Verification items for the finished model (mm, model axes). Round coordinates to 2 decimals unless told otherwise and drop trailing zeros. Loops run counter-clockwise (first coordinate to the right, second up) from the corner with the lowest first, then second, coordinate; pieces in that order, holes last. Notation, with made-up numbers: M -2,-39.75 L 2,-39.75 A20 cw 2,-6.75 Z; hole C 89.25,62.5 d7. An arc over 180 degrees is marked long. Write item = value, one per line. Start each with the question number.
from build123d import *

# Parameters (mm, degrees)
F0_R     = 3.175
F1_DEPTH = 3.048


with BuildPart() as f1:
    # F0 (on Front) → F1 (new body)
    with BuildSketch(Plane.XZ):
        with BuildLine():
            ThreePointArc((-9.525, 114.3), (0, 104.775), (9.525, 114.3))
            ThreePointArc((9.525, 114.3), (0, 123.825), (-9.525, 114.3))
        make_face()
        with Locations((0, 114.3)):
            Circle(F0_R, mode=Mode.SUBTRACT)
        with BuildLine():
            Line((15.3865384615, 67.4076923077), (9.525, 114.3))
            ThreePointArc((9.525, 114.3), (0, 104.775), (-9.525, 114.3))
            Line((-9.525, 114.3), (-15.3865384615, 67.4076923077))
            ThreePointArc((-15.3865384615, 67.4076923077), (0, 79.375), (15.3865384615, 67.4076923077))
        make_face()
        with Locations((-3.175, 99.886942851)):
            Circle(F0_R, mode=Mode.SUBTRACT)
        with BuildLine():
            Line((15.875, 63.5), (15.3865384615, 67.4076923077))
            ThreePointArc((15.3865384615, 67.4076923077), (0, 79.375), (-15.3865384615, 67.4076923077))
            Line((-15.3865384615, 67.4076923077), (-15.875, 63.5))
            Line((-15.875, 63.5), (-15.5606435644, 60.3564356436))
            ThreePointArc((-15.5606435644, 60.3564356436), (1.5796215395, 47.7037846054), (15.875, 63.5))
        make_face()
        with Locations((0, 63.5)):
            Circle(F0_R, mode=Mode.SUBTRACT)
        with BuildLine():
            ThreePointArc((15.875, 63.5), (15.7524112928, 65.4690514116), (15.3865384615, 67.4076923077))
            Line((15.3865384615, 67.4076923077), (15.875, 63.5))
        make_face()
        with BuildLine():
            Line((-15.875, 63.5), (-15.3865384615, 67.4076923077))
            ThreePointArc((-15.3865384615, 67.4076923077), (-15.7524112928, 65.4690514116), (-15.875, 63.5))
        make_face()
        with BuildLine():
            Line((15.875, 16.6322472884), (15.875, 63.5))
            ThreePointArc((15.875, 63.5), (1.5796215395, 47.7037846054), (-15.5606435644, 60.3564356436))
            Line((-15.5606435644, 60.3564356436), (-9.525, 0))
            ThreePointArc((-9.525, 0), (0, 9.525), (9.525, 0))
            ThreePointArc((9.525, 0), (6.8547876682, -6.6134341324), (0.3412706511, -9.5188843539))
            Line((0.3412706511, -9.5188843539), (44.45, -7.9375))
            ThreePointArc((44.45, -7.9375), (36.5125, 0), (44.45, 7.9375))
            Line((44.45, 7.9375), (23.5403527632, 8.6871518144))
            ThreePointArc((23.5403527632, 8.6871518144), (18.1037372263, 11.1122342659), (15.875, 16.6322472884))
        make_face()
        with BuildLine():
            Line((-15.5606435644, 60.3564356436), (-15.875, 63.5))
            ThreePointArc((-15.875, 63.5), (-15.7962153946, 61.9203784605), (-15.5606435644, 60.3564356436))
        make_face()
        with BuildLine():
            ThreePointArc((9.525, 0), (0, 9.525), (-9.525, 0))
            ThreePointArc((-9.525, 0), (-6.6134341324, -6.8547876682), (0.3412706511, -9.5188843539))
            ThreePointArc((0.3412706511, -9.5188843539), (6.8547876682, -6.6134341324), (9.525, 0))
        make_face()
        Circle(F0_R, mode=Mode.SUBTRACT)
        with BuildLine():
            ThreePointArc((52.3875, 0), (50.0626600757, 5.6126600757), (44.45, 7.9375))
            ThreePointArc((44.45, 7.9375), (36.5125, 0), (44.45, -7.9375))
            ThreePointArc((44.45, -7.9375), (50.0626600757, -5.6126600757), (52.3875, 0))
        make_face()
        with Locations((44.45, 0)):
            Circle(F0_R, mode=Mode.SUBTRACT)
    extrude(amount=F1_DEPTH)


solid = f1.part
1. Section check B-B, the plane x = 12.5. Enter the section's corners in (y, z), and give its area (3 significant figures).
2. Section check A-A, the plane y = -1.9. Give the number of separate pieces and of enclosed holes in the cut face, and give its area (3 significant figures).
3. Gauge pin test, flat ends, axial feed: P1, Ø8.5, axis at x = -3.18, z = 99.89, coming from the +Y side; P2, Ø1.5, axis at x = 13, y = -2.5, coming from the -Z side. Record the tip position at first contact, or that the pin passes through.
4. Thickness scan on line 1 (X direction, y = -1.3, z = -2.5); line 2 (X direction, y = -1.65, z = -1); line 3 (X direction, y = -0.95, z = 61) (3 decimals). Record the ranges inside material, lowest first.
5. Mould release check, pull along X, two halves, no side actions. Record for faces 1 (the cylindrical face through (41.28, -1.5, 0.14)), 2 (the flat face through (-12.585, -1.503, 30.601)), 3 (the cylindrical face through (-0.69, -1.5, -3.1)), 4 (the flat face through (15.875, -2, 40)): pulls with the +X half, pulls with the -X half, needs draft (parallel to the pull), parting line crosses it, or undercut.
6. Section check C-C, the plane z = 21. Enter the section's corners in (x, y) (3 decimals), and give its area (3 significant figures).
Computed values:
q1.outline = M -3.05,-9.08 L 0,-9.08 L 0,90.5 L -3.05,90.5 Z
q1.area = 304 mm2
q2.separate_pieces = 1
q2.enclosed_holes = 5
q2.area = 3,900 mm2
q3.P1 = 0
q3.P2 = -9.09
q4.line_1 = -9.19 to -1.96, 1.96 to 42.49, 46.41 to 51.98
q4.line_2 = -9.47 to -3.01, 3.01 to 41.44, 47.46 to 52.32
q4.line_3 = -15.677 to -1.957, 1.957 to 15.875
q5.face_1 = undercut
q5.face_2 = pulls with the -X half
q5.face_3 = undercut
q5.face_4 = pulls with the +X half
q6.outline = M -11.625,-3.048 L 15.875,-3.048 L 15.875,0 L -11.625,0 Z
q6.area = 83.8 mm2
